Here's how the part is built. I have some questions about the finished solid (model axes, mm). A direction names the side the tool comes from. Round coordinates to 2 decimals unless told otherwise and drop trailing zeros. Write each loop counter-clockwise with the first axis right and the second up, starting at its lowest first coordinate (ties: lowest second). Pieces come first, ordered by that corner, then holes. Notation, with made-up numbers: (64.25, 60) -> (93.25, 60) arc R30 ccw to (93.25, 89) -> close; hole circle Ø4 at (86, 0.25). An arc over 180 degrees is marked (long way). Answer as CSV lines item,"result".
from build123d import *

# Parameters (mm, degrees)
EXTRUDE_1_DEPTH     = 40
SKETCH_2_R          = 1.35
CUT_EXTRUDE_1_DEPTH = 1
SKETCH_3_R          = 1.35
CUT_EXTRUDE_2_DEPTH = 40


with BuildPart() as part:
    # 草图1 → 凸台-拉伸1 (new body)
    with BuildSketch(Plane.XY):
        Polygon((0, 0), (15, 0), (15, 6), (21.660254038, -5.535898385), (15.660254038, -9), (0, -9), align=None)
    extrude(amount=EXTRUDE_1_DEPTH)

    # 草图2 → 切除-拉伸1 (cut)
    with BuildSketch(Plane(origin=(13.848076211, 7.995190528, 0), x_dir=(0, 0, -1), z_dir=(0.8660254037844386, 0.4999999999999999, 0))):
        with Locations(Location((-5, -8.30384758, 0), (0, 0, 90))):
            Circle(SKETCH_2_R)
    cut_extrude_1 = extrude(amount=-CUT_EXTRUDE_1_DEPTH, mode=Mode.SUBTRACT)

    # 镜向1: 切除-拉伸1 across plane
    add(cut_extrude_1.mirror(Plane.XY.offset(20)), mode=Mode.SUBTRACT)

    # 草图3 → 切除-拉伸2 (cut)
    with BuildSketch(Plane.XY.offset(40)):
        with Locations((3, -4.5)):
            Circle(SKETCH_3_R)
        with Locations((13, -4.5)):
            Circle(SKETCH_3_R)
    extrude(amount=-CUT_EXTRUDE_2_DEPTH, mode=Mode.SUBTRACT)


solid = part.part
Item 1: Suppose I cut it at A-A, the plane x = 3. List the corners of the cut face in (y, z) for me, then the cut area to 3 significant figures.
Results found:
outline,"(-9, 0) -> (-5.85, 0) -> (-5.85, 40) -> (-9, 40) -> close; (-3.15, 0) -> (0, 0) -> (0, 40) -> (-3.15, 40) -> close"
area,"252 mm²"
Item 2: Suppose I cut it at B-B, the plane z = 30.5. List the corners of the cut face in (x, y) for me.
Results found:
outline,"(0, -9) -> (15.66, -9) -> (21.66, -5.54) -> (15, 6) -> (15, 0) -> (0, 0) -> close; hole circle Ø2.7 at (3, -4.5); hole circle Ø2.7 at (13, -4.5)"
Item 3: Will these pins go through, and if not, where does the flat tip stop? pin 1 (1.6 mm diameter, centred on x = 3, y = -4.5, fed in from +Z); pin 2 (2 mm diameter, centred on x = 4, z = 11, fed in from +Y).
Results found:
pin 1,"passes through"
pin 2,"stops at y = 0"
Item 4: I need wall thicknesses on L1, parallel to Y at x = 3, z = 23; L2, parallel to Y at x = 7.25, z = 25; L3, parallel to X at y = -3.75, z = 37.5. Which ranges of each line are inside material? Lowest first, please.
Results found:
L1,"y = -9 to -5.85, -3.15 to 0"
L2,"y = -9 to 0"
L3,"x = 0 to 1.88, 4.12 to 11.88, 14.12 to 20.63"
Item 5: For faces 4 (the flat face through (11, -5, 0)), 5 (the flat face through (15, 3, 20)), 6 (the flat face through (17.14, 0.29, 5.02)), which set-ups out of +Z, -Z, +X, -X, +Y, -Y let a thin tool reach every point of the face, with its end or its side?
Results found:
face 4,"-Z, +X, -X, +Y, -Y"
face 5,"+Z, -Z, -X, +Y"
face 6,"none"
Item 6: If we mould it in two halves opening along Z, with no side actions, what happens to faces 1 (the flat face through (17.14, 0.29, 34.98)), 2 (the flat face through (11, -5, 40)), 3 (the cylindrical face through (3.62, -5.7, 20.28))? For each: pulls with the +Z half, pulls with the -Z half, needs draft (parallel to the pull), parting line crosses it, or undercut.
Results found:
face 1,"undercut"
face 2,"pulls with the +Z half"
face 3,"needs draft"
Item 7: Suppose I cut it at C-C, the plane y = -4.5. List the corners of the cut face in (x, z) for me, then the cut area to 3 significant figures.
Results found:
outline,"(0, 0) -> (1.65, 0) -> (1.65, 40) -> (0, 40) -> close; (4.35, 0) -> (11.65, 0) -> (11.65, 40) -> (4.35, 40) -> close; (14.35, 0) -> (21.06, 0) -> (21.06, 40) -> (14.35, 40) -> close"
area,"626 mm²"
Item 8: Suppose I cut it at D-D, the plane y = -2. List the corners of the cut face in (x, z) for me, then the cut area to 3 significant figures.
Results found:
outline,"(0, 0) -> (19.62, 0) -> (19.62, 40) -> (0, 40) -> close"
area,"785 mm²"
